Work out the finished part from the listing and answer in its coordinate system (mm). A direction names the side the tool comes from. Give positions to 0.01 mm unless a question says otherwise; leave off trailing zeros. Loops run counter-clockwise (first coordinate to the right, second up) from the corner with the lowest first, then second, coordinate; pieces in that order, holes last.
```python
from build123d import *

# Parameters (mm, degrees)
F0_R     = 50
F1_DEPTH = 5
F2_R     = 50
F2_R_2   = 47.5
F3_DEPTH = 50
F4_R     = 22.5
F6_DEPTH = 55.001


# Not quite as in the source:
# - the program builds the solid bodies; features that only make, move or delete a surface that nothing else refers to are left out


with BuildPart() as f1:
    # F0 (on Front) → F1 (new body)
    with BuildSketch(Plane.XZ):
        Circle(F0_R)
    extrude(amount=-F1_DEPTH)

    # F2 (on Front) → F3 (join)
    with BuildSketch(Plane.XZ):
        Circle(F2_R)
        Circle(F2_R_2, mode=Mode.SUBTRACT)
    extrude(amount=F3_DEPTH)

    # F4 (on face) → F6 (cut, through all)
    with BuildSketch(Plane(origin=(0, 5, 0), x_dir=(-1, 0, 0), z_dir=(0, 1, 0))):
        Circle(F4_R)
    extrude(amount=-F6_DEPTH, mode=Mode.SUBTRACT)


solid = f1.part
```
Q1. Determine the mould class of faces 3 (the face through (44.2, -50, -18.3)), 4 (the face through (-10.3, -24.65, -46.37)) for opening direction Z: +Z half, -Z half, draft (parallel to the pull), parting line (faces both ways), or undercut.
Q2. Section C-C on y = -34 is taken. Give the vertices of the cut face in (x, z).
Q3. Given pin 1 (2 mm diameter, centred on y = -25, z = -33, fed in from +X); pin 2 (4 mm diameter, centred on y = -9.5, z = -18.5, fed in from -X); pin 3 (10 mm diameter, centred on x = -10, y = -23, fed in from -Z), each flat-ended and moving along its own axis, determine where each tip first touches the part or whether it passes through.
Q4. Section B-B on z = 0 is taken. Give the vertices of the cut face in (x, y).
Q5. Section A-A on x = 0 is taken. Give the vertices of the cut face in (y, z), plus the area to 3 significant figures.
Q6. Which of the six approach directions +Z, -Z, +X, -X, +Y, -Y give full straight-line access (tool end or side, diameter ignored) to faces 1 (the face through (10, 5, -22)), 2 (the face through (20.4, 0, -9.9))?
Q7. Section D-D on z = -38 is taken. Give the vertices of the cut face in (x, y).
Q8. Consider line 1 along Z through (x, y) = (0, -11); line 2 along Z through (x, y) = (0, 1); line 3 along Y through (x, z) = (-20, -14.5). Determine where each line is inside the solid, lowest interval first.
Check result:
1. face 3: draft
1. face 4: undercut
2. outline: circle Ø100 at (0, 0); hole circle Ø95 at (0, 0)
3. pin 1: stops at x = 38.42
3. pin 2: stops at x = -47.2
3. pin 3: stops at z = -49.75
4. outline: (-50, -50) - (-47.5, -50) - (-47.5, 0) - (-22.5, 0) - (-22.5, 5) - (-50, 5) - close; (22.5, 0) - (47.5, 0) - (47.5, -50) - (50, -50) - (50, 5) - (22.5, 5) - close
5. outline: (-50, -50) - (5, -50) - (5, -22.5) - (0, -22.5) - (0, -47.5) - (-50, -47.5) - close; (-50, 47.5) - (0, 47.5) - (0, 22.5) - (5, 22.5) - (5, 50) - (-50, 50) - close
5. area: 525 mm2
6. face 1: +Z, -Z, +X, -X, +Y
6. face 2: -Y
7. outline: (-32.5, -50) - (-28.5, -50) - (-28.5, 0) - (28.5, 0) - (28.5, -50) - (32.5, -50) - (32.5, 5) - (-32.5, 5) - close
8. line 1: z = -50 to -47.5, 47.5 to 50
8. line 2: z = -50 to -22.5, 22.5 to 50
8. line 3: y = 0 to 5
